```python
from build123d import *

# Parameters (mm, degrees)
SKETCH_1_R          = 10
SKETCH_1_R_2        = 1.5
EXTRUDE_1_DEPTH     = 2
SKETCH_2_R          = 4.5
SKETCH_2_R_2        = 2.75
EXTRUDE_2_DEPTH     = 2.5
SKETCH_3_R          = 2.75
CUT_EXTRUDE_1_DEPTH = 15.361406616


with BuildPart() as part:
    # 草图1 → 凸台-拉伸1 (new body)
    with BuildSketch(Plane(origin=(0, 0, 0), x_dir=(1, 0, 0), z_dir=(0, 1, 0))):
        with Locations(Location((0, 0, 0), (0, 0, 270))):
            Circle(SKETCH_1_R)
        with Locations(Location((0, 7, 0), (0, 0, 270))):
            Circle(SKETCH_1_R_2, mode=Mode.SUBTRACT)
        with Locations(Location((-7, 0, 0), (0, 0, 270))):
            Circle(SKETCH_1_R_2, mode=Mode.SUBTRACT)
        with Locations(Location((0, -7, 0), (0, 0, 270))):
            Circle(SKETCH_1_R_2, mode=Mode.SUBTRACT)
        with Locations(Location((7, 0, 0), (0, 0, 270))):
            Circle(SKETCH_1_R_2, mode=Mode.SUBTRACT)
    extrude(amount=EXTRUDE_1_DEPTH)

    # 草图2 → 凸台-拉伸2 (add)
    with BuildSketch(Plane(origin=(0, 2, 0), x_dir=(1, 0, 0), z_dir=(0, 1, 0))):
        with Locations(Location((0, 0, 0), (0, 0, 270))):
            Circle(SKETCH_2_R)
        with Locations(Location((0, 0, 0), (0, 0, 270))):
            Circle(SKETCH_2_R_2, mode=Mode.SUBTRACT)
    extrude(amount=EXTRUDE_2_DEPTH)

    # 草图3 → 切除-拉伸1 (cut, through all)
    with BuildSketch(Plane(origin=(0, 2, 0), x_dir=(1, 0, 0), z_dir=(0, 1, 0))):
        with Locations(Location((0, 0, 0), (0, 0, 270))):
            Circle(SKETCH_3_R)
    extrude(amount=-CUT_EXTRUDE_1_DEPTH, mode=Mode.SUBTRACT)


solid = part.part
```
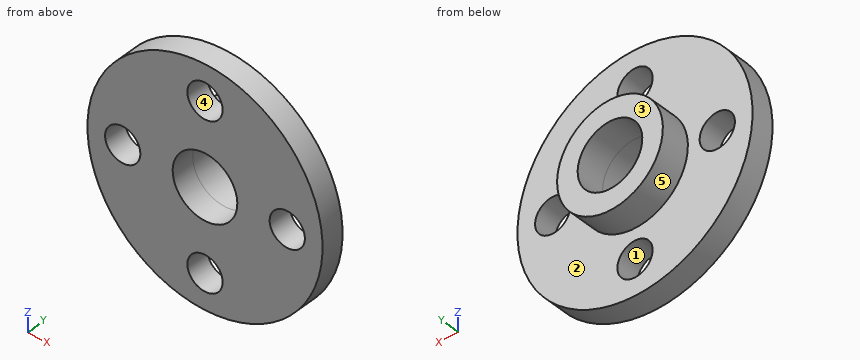
Here's how the part is built. I have some questions about the finished solid (model axes, mm). Face numbers are marked on the shaded views. A direction names the side the tool comes from. Give positions to 0.01 mm unless a question says otherwise; leave off trailing zeros. Loops run counter-clockwise (first coordinate to the right, second up) from the corner with the lowest first, then second, coordinate; pieces in that order, holes last. Notation, with made-up numbers: M 43.5,-1 L 51.5,-1 A33 cw 51.5,34 Z; hole C -10.5,-11 d1. An arc over 180 degrees is marked long. Use one line per item in the form item = value. Start each with the question number.
Q1. Thinking about a two-plate mould opening in Z: for the marked faces 3, 4 and 5, which applies, +Z half, -Z half, draft (parallel to the pull), parting line (faces both ways), or undercut?
Q2. If we section it at B-B (x = 0): Write out the boundary of the cut face in (y, z), then the cut area to 4 significant figures.
Q3. I need wall thicknesses on line 1 along X through (y, z) = (1.65, 0); line 2 along Z through (x, y) = (-1, 0.9); line 3 along X through (y, z) = (1.15, 0.5). Which ranges of each line are inside material? Lowest first, please.
Q4. Will these pins go through, and if not, where does the flat tip stop? pin 1 Ø3 at (x, z) = (-1.5, 1) entering from +Y; pin 2 Ø1 at (y, z) = (2, 6) entering from +X.
Q5. If we section it at D-D (x = -7): Write out the boundary of the cut face in (y, z), then the cut area to 3 significant figures.
Q6. If we section it at C-C (y = 0.85): Write out the boundary of the cut face in (x, z).
Q7. Which directions (+Z, -Z, +X, -X, +Y, -Y) give clear straight access to the entire face, cutting with the end or side of a thin tool? Please do the marked faces 1 and 2.
Q8. If we section it at A-A (z = 0): Write out the boundary of the cut face in (x, y).
Taken from the geometry:
q1.face_3 = draft
q1.face_4 = undercut
q1.face_5 = parting line
q2.outline = M 0,-10 L 2,-10 L 2,-8.5 L 0,-8.5 Z; M 0,-5.5 L 2,-5.5 L 2,-4.5 L 4.5,-4.5 L 4.5,-2.75 L 0,-2.75 Z; M 0,2.75 L 4.5,2.75 L 4.5,4.5 L 2,4.5 L 2,5.5 L 0,5.5 Z; M 0,8.5 L 2,8.5 L 2,10 L 0,10 Z
q2.area = 25.75 mm^2
q3.line_1 = -10 to -8.5, -5.5 to -2.75, 2.75 to 5.5, 8.5 to 10
q3.line_2 = -9.95 to -8.12, -5.88 to -2.56, 2.56 to 5.88, 8.12 to 9.95
q3.line_3 = -9.99 to -8.41, -5.59 to -2.7, 2.7 to 5.59, 8.41 to 9.99
q4.pin_1 = 4.5
q4.pin_2 = 8.35
q5.outline = M 0,-7.14 L 2,-7.14 L 2,-1.5 L 0,-1.5 Z; M 0,1.5 L 2,1.5 L 2,7.14 L 0,7.14 Z
q5.area = 22.6 mm^2
q6.outline = C 0,0 d20; hole C -7,0 d3; hole C 0,0 d5.5; hole C 0,-7 d3; hole C 0,7 d3; hole C 7,0 d3
q7.face_1 = +Y, -Y
q7.face_2 = +Y
q8.outline = M -10,0 L -8.5,0 L -8.5,2 L -10,2 Z; M -5.5,0 L -2.75,0 L -2.75,4.5 L -4.5,4.5 L -4.5,2 L -5.5,2 Z; M 2.75,0 L 5.5,0 L 5.5,2 L 4.5,2 L 4.5,4.5 L 2.75,4.5 Z; M 8.5,0 L 10,0 L 10,2 L 8.5,2 Z
